Design review of the part built by this model. Coordinates are the model's own, in mm. A direction names the side the tool comes from. Give positions to 0.01 mm unless a question says otherwise; leave off trailing zeros. Loops run counter-clockwise (first coordinate to the right, second up) from the corner with the lowest first, then second, coordinate; pieces in that order, holes last.
from build123d import *

# Parameters (mm, degrees)
F2_R     = 2.75
F3_DEPTH = 60
F4_R     = 2.75
F5_DEPTH = 60


with BuildPart() as f1:
    # F0 (on Front) → F1 (revolve)
    with BuildSketch(Plane.XZ):
        with BuildLine():
            Line((-37.5, 40), (-37.5, 0))
            Line((-37.5, 0), (-31.5, 0))
            Line((-31.5, 0), (-31.5, 37.5))
            ThreePointArc((-31.5, 37.5), (-16.943087, 46.756579), (0, 50))
            Line((0, 50), (0, 55.5))
            ThreePointArc((0, 55.5), (-20.393033, 51.72508), (-37.5, 40))
        make_face()
    revolve(axis=Axis((0, 0, -14.908669), (0, 0, -1)))

    # F2 (on Top) → F3 (cut)
    with BuildSketch(Plane.XY):
        Circle(F2_R)
    extrude(amount=F3_DEPTH, mode=Mode.SUBTRACT)

    # F4 (on Top) → F5 (cut)
    with BuildSketch(Plane.XY):
        with Locations((11, 0)):
            Circle(F4_R)
    extrude(amount=F5_DEPTH, mode=Mode.SUBTRACT)


solid = f1.part
Q1. Wall thickness on line 1 (X direction, y = 0, z = 51.5); line 2 (X direction, y = 0, z = 50.5); line 3 (Y direction, x = 0, z = 20.5): over which ranges is each line inside the solid? List them lowest first.
Results:
line 1: x = -20.93 to -2.75, 2.75 to 8.25, 13.75 to 20.93
line 2: x = -23.12 to -2.75, 2.75 to 8.25, 13.75 to 23.12
line 3: y = -37.5 to -31.5, 31.5 to 37.5
Q2. Tool access review of faces 4 (the face through (-0.596, -2.685, 52.667)), 5 (the face through (4.101, 31.232, 19.012)): name each direction out of +Z, -Z, +X, -X, +Y, -Y from which nothing blocks a thin tool from reaching the whole face with its end or side.
Results:
face 4: +Z, -Z
face 5: -Z
Q3. Insertion check: pin 1 (2 mm diameter, centred on x = -13, z = 42, fed in from +Y); pin 2 (3 mm diameter, centred on x = 18, y = -20.5, fed in from +Z); pin 3 (6 mm diameter, centred on x = -18, y = 3.5, fed in from -Z); pin 4 (3.5 mm diameter, centred on x = 11, y = 0, fed in from +Z). Each pin has a flat end and moves straight along its axis. Give the tip position at first contact, or say it passes through.
Results:
pin 1: stops at y = 34.19
pin 2: stops at z = 49.11
pin 3: stops at z = 44.74
pin 4: passes through
Q4. Take a section at A-A (z = 4). Give the boundary of the cut face in (x, y), plus the area to 3 significant figures.
Results:
outline: circle Ø75 at (0, 0); hole circle Ø63 at (0, 0)
area: 1,300 mm2
Q5. Take a section at B-B (y = 0). Give the number of separate pieces and of enclosed holes in the cut face, plus the area to 3 significant figures.
Results:
separate pieces: 3
enclosed holes: 0
area: 850 mm2
Q6. Draft analysis for pull direction X (two halves, no side actions). For faces 1 (the face through (13.54, -1.05, 51.41)), 2 (the face through (9, 31, 0)), 3 (the face through (4.88, 37.18, 19.72)), state which applies: pulls with the +X half, pulls with the -X half, needs draft (parallel to the pull), parting line crosses it, or undercut.
Results:
face 1: undercut
face 2: needs draft
face 3: parting line crosses it
